from build123d import *

# Parameters (mm, degrees)
CROQUIS1_R              = 1.475
SALIENTE_EXTRUIR1_DEPTH = 27
CHAFL_N1_SIZE           = 0.5
CHAFL_N1_SIZE2          = 0.288675135
CHAFL_N7_SIZE           = 0.5
CHAFL_N7_SIZE2          = 0.595876796


with BuildPart() as part:
    # Croquis1 → Saliente-Extruir1 (new body)
    with BuildSketch(Plane(origin=(0, 0, 0), x_dir=(0, 0, -1), z_dir=(1, 0, 0))):
        Circle(CROQUIS1_R)
    extrude(amount=SALIENTE_EXTRUIR1_DEPTH)

    # Chaflán1
    chafl_n1_edges = [part.edges().sort_by_distance(p)[0] for p in [
        (27, 0, 1.475),
    ]]
    chafl_n1_side = [part.faces().sort_by_distance(p)[0] for p in [
        (13.5, 0, 1.475),
    ]]
    chamfer(chafl_n1_edges, length=CHAFL_N1_SIZE, length2=CHAFL_N1_SIZE2, reference=chafl_n1_side[0])

    # Chaflán7
    chafl_n7_edges = [part.edges().sort_by_distance(p)[0] for p in [
        (0, 0, 1.475),
    ]]
    chafl_n7_side = [part.faces().sort_by_distance(p)[0] for p in [
        (0, 0, 0),
    ]]
    chamfer(chafl_n7_edges, length=CHAFL_N7_SIZE, length2=CHAFL_N7_SIZE2, reference=chafl_n7_side[0])


solid = part.part
The listing builds one solid part. Answer for the finished solid, in the listing's coordinates (mm). Coordinates: 2 decimals unless noted, no trailing zeros. Write each loop counter-clockwise with the first axis right and the second up, starting at its lowest first coordinate (ties: lowest second). Pieces come first, ordered by that corner, then holes. Notation, with made-up numbers: (64, 11.25) -> (110, 11.25) arc R22 ccw to (110, 38.25) -> close; hole circle Ø9 at (58, 71). An arc over 180 degrees is marked (long way). One line per question, with ' | ' between items.
1. Straight lines are drawn through the part: line 1 (Y direction, x = 6, z = -0.75); line 2 (Y direction, x = 8, z = 1.2); line 3 (X direction, y = 0.3, z = -1.1). For each, find the intervals that lie inside material, in ascending order.
Verdict:
line 1: y = -1.27 to 1.27 | line 2: y = -0.86 to 0.86 | line 3: x = 0.2 to 27
2. Given pin 1 Ø1 at (x, z) = (22.5, 1) entering from +Y, flat-ended and moving along its own axis, determine where the tip first touches the part or whether it passes through.
Verdict:
pin 1: stops at y = 1.39
3. Section A-A (x = 7) is taken. Determine the outline of the cut face in (y, z) (3 decimals), and give its area (3 significant figures).
Verdict:
outline: circle Ø2.95 at (0, 0) | area: 6.83 mm^2
